from build123d import *

# Parameters (mm, degrees)
SKETCH1_W          = 21.06
SKETCH1_H          = 15.8
EXTRUDE1_DEPTH     = 13.06
SKETCH2_R          = 1.5
EXTRUDE2_DEPTH     = 3.25
CUT_EXTRUDE1_DEPTH = 18


with BuildPart() as part:
    # Sketch1 → Extrude1 (new body)
    with BuildSketch(Plane.XY):
        with Locations((10.53, -7.9)):
            Rectangle(SKETCH1_W, SKETCH1_H)
    extrude(amount=EXTRUDE1_DEPTH)

    # Sketch2 → Extrude2 (add)
    with BuildSketch(Plane(origin=(0, 0, 0), x_dir=(-1, 0, 0), z_dir=(0, 0, -1))):
        with Locations((-10.34, -2.25)):
            Circle(SKETCH2_R)
        with Locations((-10.34, -13.68)):
            Circle(SKETCH2_R)
    extrude(amount=EXTRUDE2_DEPTH)

    # Sketch3 → Cut-Extrude1 (cut)
    with BuildSketch(Plane(origin=(21.06, 0, 0), x_dir=(0, 0, -1), z_dir=(1, 0, 0))):
        Polygon((-11.809509458, -14.113172182), (-11.809509458, -1.403202269), (-2.254873777, -1.403202269), (-2.254873777, -5.498046132), (-0.819019435, -5.498046132), (-0.819019435, -9.858788948), (-2.254873777, -9.858788948), (-2.254873777, -14.113172182), align=None)
    extrude(amount=-CUT_EXTRUDE1_DEPTH, mode=Mode.SUBTRACT)


solid = part.part
Model file for the job. Use its own axes, mm. A direction names the side the tool comes from. Give positions to 0.01 mm unless a question says otherwise; leave off trailing zeros. Order: outer loops, then holes, each group sorted by start corner. A loop starts at its lowest first (then second) coordinate and runs counter-clockwise, first axis right, second up. Notation, with made-up numbers: M 19,-32 L 29,-32 A20 cw 29,3 Z; hole C 72,33.5 d3. An arc over 180 degrees is marked long. Write item = value, one per line.
Q1. Drill centre lines: line 1 (Y direction, x = 18, z = 10.5); line 2 (Z direction, x = 20.25, y = -8.25); line 3 (Y direction, x = 12.75, z = 1). Where is each one in solid material? Low to high. Write a range as [from, to].
Derived:
line_1 = [-15.8, -14.11], [-1.4, 0]
line_2 = [0, 0.82], [11.81, 13.06]
line_3 = [-15.8, -9.86], [-5.5, 0]
Q2. Cut at C-C, the plane z = 6. List the corners of the cut face in (x, y), then the cut area to 3 significant figures.
Derived:
outline = M 0,-15.8 L 21.06,-15.8 L 21.06,-14.11 L 3.06,-14.11 L 3.06,-1.4 L 21.06,-1.4 L 21.06,0 L 0,0 Z
area = 104 mm2
Q3. Cut at D-D, the plane x = 19.5. List the corners of the cut face in (y, z), then the cut area to 3 significant figures.
Derived:
outline = M -15.8,0 L 0,0 L 0,13.06 L -15.8,13.06 Z; hole M -14.11,2.25 L -9.86,2.25 L -9.86,0.82 L -5.5,0.82 L -5.5,2.25 L -1.4,2.25 L -1.4,11.81 L -14.11,11.81 Z
area = 78.6 mm2
Q4. Cut at A-A, the plane x = 10.34. List the corners of the cut face in (y, z), then the cut area to 3 significant figures.
Derived:
outline = M -15.8,0 L -15.18,0 L -15.18,-3.25 L -12.18,-3.25 L -12.18,0 L -3.75,0 L -3.75,-3.25 L -0.75,-3.25 L -0.75,0 L 0,0 L 0,13.06 L -15.8,13.06 Z; hole M -14.11,2.25 L -9.86,2.25 L -9.86,0.82 L -5.5,0.82 L -5.5,2.25 L -1.4,2.25 L -1.4,11.81 L -14.11,11.81 Z
area = 98.1 mm2
Q5. Cut at B-B, the plane y = -9. List the corners of the cut face in (x, z), then the cut area to 3 significant figures.
Derived:
outline = M 0,0 L 21.06,0 L 21.06,0.82 L 3.06,0.82 L 3.06,11.81 L 21.06,11.81 L 21.06,13.06 L 0,13.06 Z
area = 77.2 mm2
Q6. Tool access for faces 5 (the flat face through (0, -8, 6)), 6 (the cylindrical face through (11.53, -14.59, -1.6)), 7 (the flat face through (12, -5.498, 2)): list every direction of +Z, -Z, +X, -X, +Y, -Y with a clear straight run to the whole face (end or side of a thin tool).
Derived:
face_5 = +Z, -Z, -X, +Y, -Y
face_6 = -Z
face_7 = +X
Q7. Two-plate mould, pull along Z, no slides. Class faces 1 (the cylindrical face through (11.84, -2.18, -1.6)), 2 (the flat face through (10, -8, 13.06)), 3 (the flat face through (12, -9.859, 2)), 4 (the flat face through (10, -2, -3.25)): pulls with the +Z half, pulls with the -Z half, needs draft (parallel to the pull), parting line crosses it, or undercut.
Derived:
face_1 = needs draft
face_2 = pulls with the +Z half
face_3 = undercut
face_4 = pulls with the -Z half
Q8. Flat gauge pins, fed straight in: pin 1 (1 mm diameter, centred on x = 12, y = -5.5, fed in from -Z); pin 2 (5.5 mm diameter, centred on y = -5, z = 8, fed in from +X). Where does each tip first touch, or does it go through?
Derived:
pin_1 = 0
pin_2 = 3.06
